Check sheet for the modelled part. Datum: model origin and axes. Units: mm. Face numbers are marked on the shaded views. A direction names the side the tool comes from. Give positions to 0.01 mm unless a question says otherwise; leave off trailing zeros. Order: outer loops, then holes, each group sorted by start corner. A loop starts at its lowest first (then second) coordinate and runs counter-clockwise, first axis right, second up. Notation, with made-up numbers: (51, -22.5) -> (58, -22.5) arc R17 ccw to (58, -14.5) -> close; hole circle Ø8 at (50, 45.5). An arc over 180 degrees is marked (long way). One line per question, with ' | ' between items.
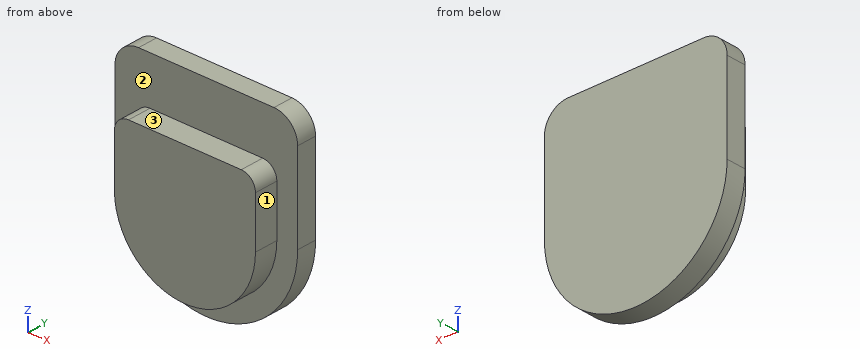
```python
from build123d import *

# Parameters (mm, degrees)
F1_DEPTH = 4.2
F3_DEPTH = 5
F4_R     = 5
F5_R     = 3


with BuildPart() as f1:
    # F0 (on Front) → F1 (new body)
    with BuildSketch(Plane.XZ):
        with BuildLine():
            Line((-19.3, 13.7), (-19.3, 0))
            ThreePointArc((-19.3, 0), (0, -19.3), (19.3, 0))
            Line((19.3, 0), (19.3, 13.7))
            Line((19.3, 13.7), (19.3, 23.7))
            Line((19.3, 23.7), (-19.3, 23.7))
            Line((-19.3, 23.7), (-19.3, 13.7))
        make_face()
    extrude(amount=-F1_DEPTH)

    # F2 (on Front) → F3 (join)
    with BuildSketch(Plane.XZ):
        with BuildLine():
            Line((-14.9, 13.7), (-14.9, 0))
            ThreePointArc((-14.9, 0), (0, -14.9), (14.9, 0))
            Line((14.9, 0), (14.9, 13.7))
            Line((14.9, 13.7), (-14.9, 13.7))
        make_face()
    extrude(amount=F3_DEPTH)

    # F4
    f4_edges = [f1.edges().sort_by_distance(p)[0] for p in [
        (-19.3, 2.1, 23.7),
        (19.3, 2.1, 23.7),
    ]]
    fillet(f4_edges, radius=F4_R)

    # F5
    f5_edges = [f1.edges().sort_by_distance(p)[0] for p in [
        (-14.9, -2.5, 13.7),
        (14.9, -2.5, 13.7),
    ]]
    fillet(f5_edges, radius=F5_R)


solid = f1.part
```
Q1. Section check C-C (y = -0.75). Enter the section's corners in (x, z).
Result sheet:
outline: (-14.9, 0) arc R14.9 ccw to (14.9, 0) -> (14.9, 10.7) arc R3 ccw to (11.9, 13.7) -> (-11.9, 13.7) arc R3 ccw to (-14.9, 10.7) -> close
Q2. Section check B-B (z = 5). Enter the section's corners in (x, y).
Result sheet:
outline: (-19.3, 0) -> (-14.9, 0) -> (-14.9, -5) -> (14.9, -5) -> (14.9, 0) -> (19.3, 0) -> (19.3, 4.2) -> (-19.3, 4.2) -> close
Q3. Depth check by flat-ended pin: pin 1 Ø2.5 at (y, z) = (-1.5, 3.5) entering from -X; pin 2 Ø4 at (x, y) = (1, -2.5) entering from +Z; pin 3 Ø1.5 at (x, y) = (13, 1) entering from -Z. Enter the tip coordinate at first touch or a pass-through.
Result sheet:
pin 1: stops at x = -14.9 | pin 2: stops at z = 13.7 | pin 3: stops at z = -14.91
Q4. Section check A-A (x = 0). Enter the section's corners in (y, z).
Result sheet:
outline: (-5, -14.9) -> (0, -14.9) -> (0, -19.3) -> (4.2, -19.3) -> (4.2, 23.7) -> (0, 23.7) -> (0, 13.7) -> (-5, 13.7) -> close
Q5. Thickness scan on line 1 (X direction, y = -3.75, z = 7.5); line 2 (Z direction, x = 0.5, y = -4.5); line 3 (X direction, y = -2.25, z = 13). Record the ranges inside material, lowest first.
Result sheet:
line 1: x = -14.9 to 14.9 | line 2: z = -14.89 to 13.7 | line 3: x = -13.83 to 13.83
Q6. Section check D-D (y = 2). Enter the section's corners in (x, z), and give its area (3 significant figures).
Result sheet:
outline: (-19.3, 0) arc R19.3 ccw to (19.3, 0) -> (19.3, 18.7) arc R5 ccw to (14.3, 23.7) -> (-14.3, 23.7) arc R5 ccw to (-19.3, 18.7) -> close | area: 1,490 mm2
Q7. Access from +Z, -Z, +X, -X, +Y, -Y to the whole of each face (thin tool, end or side, straight path). Record for the marked faces 1, 2 and 3.
Result sheet:
face 1: +Z, -Z, +X, -Y | face 2: -Y | face 3: +Z, +X, -X, -Y
